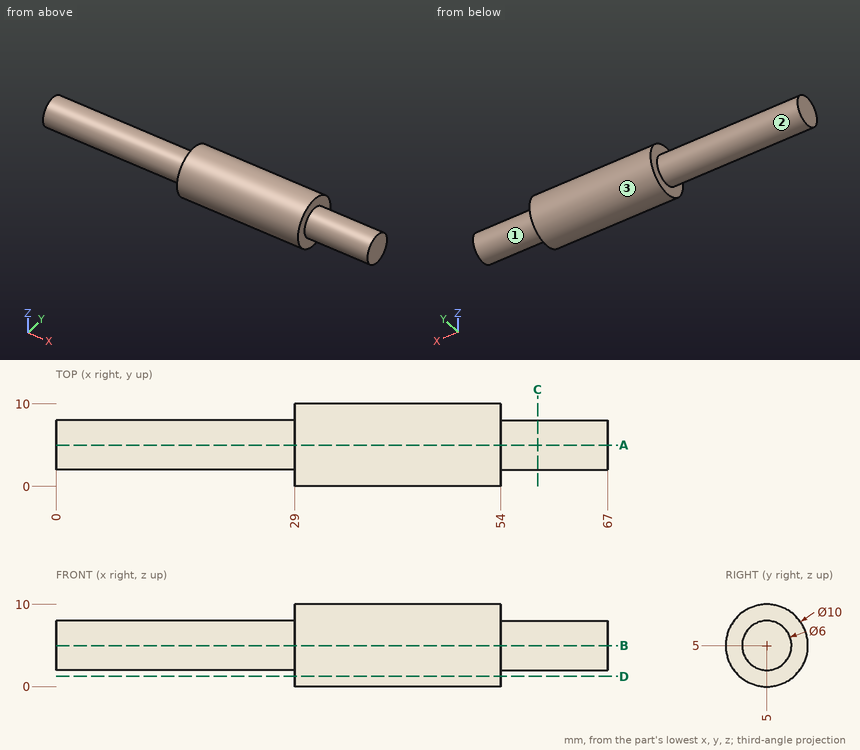
Answer from the drawing. Dimensions are ordinates in mm from the lowest x, y and z of the part. A direction names the side the tool comes from. Round coordinates to 2 decimals unless told otherwise and drop trailing zeros. Loops run counter-clockwise (first coordinate to the right, second up) from the corner with the lowest first, then second, coordinate; pieces in that order, holes last. Notation, with made-up numbers: (-39, -25.75) - (16, -25.75) arc R24 cw to (16, -9.75) - close; hole circle Ø9 at (-14.75, 85.25). An arc over 180 degrees is marked (long way). Return JSON: item names as keys, results as strings. Group by question number.
1. The part is cut by section D-D on z = 1.25. Determine the outline of the cut face in (x, y), then the cut area to 3 significant figures.
2. Which of the six approach directions +Z, -Z, +X, -X, +Y, -Y give full straight-line access (tool end or side, diameter ignored) to the marked faces 1, 2 and 3?
3. The part is cut by section C-C on x = 58.5. Determine the outline of the cut face in (y, z), then the cut area to 3 significant figures.
4. Consider probe 1 along X at (y, z) = (8, 4.25); probe 2 along Z at (x, y) = (42, 1); probe 3 along Y at (x, z) = (30.5, 4.75). Determine where each line is inside the solid, lowest interval first.
5. Each of these flat-tipped pins is pushed along its axis until it touches: P1, Ø2, axis at x = 17.5, z = 6.5, coming from the +Y side; P2, Ø1, axis at x = 26, z = 5, coming from the -Y side; P3, Ø2, axis at x = 24.5, y = 2, coming from the -Z side; P4, Ø5, axis at y = 9, z = 3.5, coming from the -X side. Where does it stop, or does it pass through?
6. The part is cut by section A-A on y = 5. Determine the outline of the cut face in (x, z), then the cut area to 3 significant figures.
Resolved:
{
 "1": {"outline": "(29, 1.69) - (54, 1.69) - (54, 8.31) - (29, 8.31) - close", "area": "165 mm²"},
 "2": {"face 1": "+X", "face 2": "-X", "face 3": "+X, -X"},
 "3": {"outline": "circle Ø6 at (5, 5)", "area": "28.3 mm²"},
 "4": {"probe 1": "x = 29 to 54", "probe 2": "z = 2 to 8", "probe 3": "y = 0.01 to 9.99"},
 "5": {"P1": "stops at y = 7.96", "P2": "stops at y = 2", "P3": "stops at z = 2.76", "P4": "stops at x = 0"},
 "6": {"outline": "(0, 2) - (29, 2) - (29, 0) - (54, 0) - (54, 2) - (67, 2) - (67, 8) - (54, 8) - (54, 10) - (29, 10) - (29, 8) - (0, 8) - close", "area": "502 mm²"}
}
